from build123d import *

# Parameters (mm, degrees)
SKETCH1_W                        = 101.6
SKETCH1_H                        = 241.3
BOSS_EXTRUDE1_DEPTH              = 19.05
TAP_DRILL_FOR_M4_HELICOIL0_D     = 4.2
TAP_DRILL_FOR_M4_HELICOIL0_DEPTH = 11.4000026
TAP_DRILL_FOR_M4_HELICOIL0_TIP   = 1.2618073


with BuildPart() as part:
    # Sketch1 → Boss-Extrude1 (new body)
    with BuildSketch(Plane(origin=(0, 4848.835870432, 0), x_dir=(1, 0, 0), z_dir=(0, 0, 1))):
        with Locations((-370.62448934, 15.409688746)):
            Rectangle(SKETCH1_W, SKETCH1_H)
    extrude(amount=BOSS_EXTRUDE1_DEPTH)

    # Tap Drill for M4 Helicoil0
    with Locations(Plane(origin=(0, 0, 19.05), x_dir=(-1, 0, 0), z_dir=(0, 0, 1))):
        with Locations((383.62448934, -4912.995559179), (357.624489341, -4912.995559179), (357.62448934, -4953.995559179), (383.62448934, -4953.995559179), (383.624489341, -4774.495559179), (383.624489341, -4815.495559179), (357.624489341, -4815.495559179), (357.62448934, -4774.495559179)):
            Hole(TAP_DRILL_FOR_M4_HELICOIL0_D / 2, depth=TAP_DRILL_FOR_M4_HELICOIL0_DEPTH)
            with Locations((0, 0, -(TAP_DRILL_FOR_M4_HELICOIL0_DEPTH + TAP_DRILL_FOR_M4_HELICOIL0_TIP / 2))):  # 118° drill point
                Cone(0, TAP_DRILL_FOR_M4_HELICOIL0_D / 2, TAP_DRILL_FOR_M4_HELICOIL0_TIP, mode=Mode.SUBTRACT)


solid = part.part
The listing builds one solid part. Answer for the finished solid, in the listing's coordinates (mm). A direction names the side the tool comes from. Round coordinates to 2 decimals unless told otherwise and drop trailing zeros. Write each question's results on one line, items separated by ' | '. Start each with the question number.
Item 1: For a pull along Y with two mould halves and no side action, classify faces 3 (the face through (-384.08, 4817.546, 13.27)), 4 (the face through (-421.424, 4863, 9)), 5 (the face through (-371, 4743.596, 9)) as pulls with the +Y half, pulls with the -Y half, needs draft (parallel to the pull), parting line crosses it, or undercut.
Item 2: For faces 1 (the face through (-371, 4866, 0)), 2 (the face through (-358.08, 4776.546, 13.27)), determine the directions among +Z, -Z, +X, -X, +Y, -Y from which every point of the face is accessible in a straight line to the end or side of a thin tool.
Item 3: A flat-ended cylindrical pin translates along its axis: pin 1 Ø3.5 at (x, y) = (-383.62, 4954) entering from +Z. Find the tip coordinate at first contact, or state that the pin passes through.
Item 4: Straight lines are drawn through the part: L1, parallel to X at y = 4954, z = 6.75; L2, parallel to Y at x = -359, z = 13.5. For each, find the intervals that lie inside material, in ascending order. Write a range as [from, to].
Check sheet entries:
1) face 3: undercut | face 4: needs draft | face 5: pulls with the -Y half
2) face 1: -Z, +X, -X, +Y, -Y | face 2: +Z
3) pin 1: z = 7.44
4) L1: [-421.42, -384.23], [-383.02, -358.23], [-357.02, -319.82] | L2: [4743.6, 4772.91], [4776.08, 4813.91], [4817.08, 4911.41], [4914.58, 4952.41], [4955.58, 4984.9]
